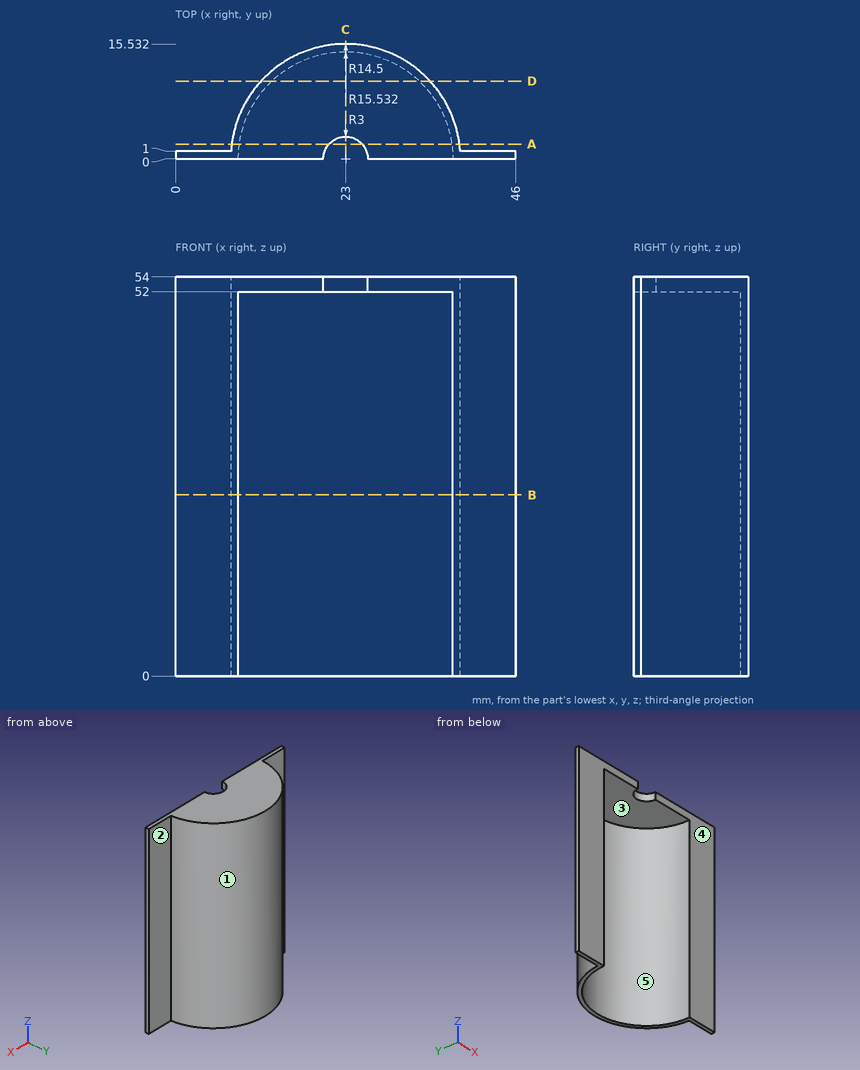
Design review of the part shown in the three views and the two pictorial views. Dimensions are in mm from the part's minimum x, y and z. A direction names the side the tool comes from. Round coordinates to 2 decimals unless told otherwise and drop trailing zeros. Write each loop counter-clockwise with the first axis right and the second up, starting at its lowest first coordinate (ties: lowest second). Pieces come first, ordered by that corner, then holes.
Item 1: The part is to be moulded in two halves that separate along X. For the marked faces 1, 2 and 3, say which applies: +X half, -X half, draft (parallel to the pull), parting line (faces both ways), or undercut.
Item 2: Clearance check with flat-ended pins moving along their axes: pin 1 Ø1 at (x, z) = (14, 35.5) entering from -Y (1 decimal); pin 2 Ø1 at (x, z) = (24, 39.5) entering from +Y; pin 3 Ø1 at (x, z) = (21, 40) entering from -Y. State where each tip first meets the part, or that it passes through.
Item 3: We need section B-B on z = 24.5. Write out the cut boundary in (x, y).
Item 4: For the marked faces 4 and 5, list the 3-axis set-ups (+Z, -Z, +X, -X, +Y, -Y) from which the entire face can be reached by the end or side of a thin tool; tool diameter is ignored.
Item 5: For probe 1 along Y at (x, z) = (23.5, 28); probe 2 along X at (y, z) = (4, 34.5); probe 3 along Y at (x, z) = (5, 40.5), list the stretches that pass through material, from the lowest coordinate up.
Item 6: We need section A-A on y = 2. Write out the cut boundary in (x, z), and give its area (3 significant figures).
Item 7: We need section D-D on y = 10.5. Write out the cut boundary in (x, z).
Item 8: We need section C-C on x = 23. Write out the cut boundary in (y, z).
Returned:
1. face 1: parting line
1. face 2: draft
1. face 3: undercut
2. pin 1: stops at y = 11
2. pin 2: stops at y = 15.52
2. pin 3: stops at y = 14.28
3. outline: (0, 0) - (8.5, 0) arc R14.5 cw to (37.5, 0) - (46, 0) - (46, 1) - (38.5, 1) arc R15.53 ccw to (7.5, 1) - (0, 1) - close
4. face 4: +Z, -Z, +X, -X, -Y
4. face 5: -Z, -Y
5. probe 1: y = 14.49 to 15.52
5. probe 2: x = 7.99 to 9.06, 36.94 to 38.01
5. probe 3: y = 0 to 1
6. outline: (7.6, 0) - (8.64, 0) - (8.64, 52) - (20.76, 52) - (20.76, 54) - (7.6, 54) - close; (25.24, 52) - (37.36, 52) - (37.36, 0) - (38.4, 0) - (38.4, 54) - (25.24, 54) - close
6. area: 161 mm2
7. outline: (11.55, 0) - (13, 0) - (13, 52) - (33, 52) - (33, 0) - (34.45, 0) - (34.45, 54) - (11.55, 54) - close
8. outline: (3, 52) - (14.5, 52) - (14.5, 0) - (15.53, 0) - (15.53, 54) - (3, 54) - close
